Check sheet for the modelled part. Datum: model origin and axes. Units: mm. A direction names the side the tool comes from. Round coordinates to 2 decimals unless told otherwise and drop trailing zeros. Order: outer loops, then holes, each group sorted by start corner. A loop starts at its lowest first (then second) coordinate and runs counter-clockwise, first axis right, second up. Notation, with made-up numbers: (47.25, -38) -> (65.25, -38) arc R31 ccw to (65.25, -9) -> close; hole circle Ø5 at (59.5, 41). An arc over 180 degrees is marked (long way). Answer in a Markdown table with one row per item.
from build123d import *

# Parameters (mm, degrees)
F1_DEPTH = 7
F2_DEPTH = 6
F3_DEPTH = 15


# Not quite as in the source:
# - a feature names something its author has since deleted; it is built from what else it names


with BuildPart() as f1:
    # F0 (on Front) → F1 (new body)
    with BuildSketch(Plane.XZ):
        with BuildLine():
            Line((-4.090710345, -1.9507641112), (-3.3236176952, -1.6008211246))
            Line((-3.3236176952, -1.6008211246), (-3.3236176952, -2.2903047641))
            Line((-3.3236176952, -2.2903047641), (-2.8842022451, -2.2903047641))
            ThreePointArc((-2.8842022451, -2.2903047641), (0.0905031972, 3.0539098469), (3.0652086395, -2.2903047641))
            Line((3.0652086395, -2.2903047641), (3.4491920394, -2.2903047641))
            Line((3.4491920394, -2.2903047641), (3.4491920394, -1.6408955531))
            Line((3.4491920394, -1.6408955531), (4.2162846892, -1.9507641112))
            Line((4.2162846892, -1.9507641112), (4.4794066601, -1.1210844752))
            ThreePointArc((4.4794066601, -1.1210844752), (4.6290079186, 0.2570213688), (4.2328723206, 1.5854162054))
            Line((4.2328723206, 1.5854162054), (5.5865912817, 3.465253188))
            Line((5.5865912817, 3.465253188), (5.5865912817, 5.931237081))
            Line((5.5865912817, 5.931237081), (1.5955031972, 5.931237081))
            Line((1.5955031972, 5.931237081), (4.5903746292, 3.397220974))
            Line((4.5903746292, 3.397220974), (0.0905031972, 3.431237081))
            Line((0.0905031972, 3.431237081), (-4.4093682348, 3.465253188))
            Line((-4.4093682348, 3.465253188), (-1.4144968028, 5.931237081))
            Line((-1.4144968028, 5.931237081), (-5.4144968028, 5.931237081))
            Line((-5.4144968028, 5.931237081), (-5.4144968028, 3.465253188))
            Line((-5.4144968028, 3.465253188), (-4.1709532845, 1.6969049432))
            ThreePointArc((-4.1709532845, 1.6969049432), (-4.6426172218, -0.138188052), (-4.090710345, -1.9507641112))
        make_face()
        Polygon((-3.3236176952, -2.2903047641), (-3.3236176952, -1.6008211246), (-4.090710345, -1.9507641112), (-4.090710345, -2.2903047641), align=None)
        with BuildLine():
            Line((-2.8842022451, -2.2903047641), (-3.3236176952, -2.2903047641))
            Line((-3.3236176952, -2.2903047641), (-4.090710345, -2.2903047641))
            Line((-4.090710345, -2.2903047641), (-4.090710345, -4.9565606735))
            Line((-4.090710345, -4.9565606735), (-3.3236176952, -4.9565606735))
            Line((-3.3236176952, -4.9565606735), (-2.590710345, -4.9565606735))
            Line((-2.590710345, -4.9565606735), (-2.590710345, -3.7436034497))
            Line((-2.590710345, -3.7436034497), (-2.590710345, -2.6957776739))
            ThreePointArc((-2.590710345, -2.6957776739), (-2.7447140714, -2.4982945873), (-2.8842022451, -2.2903047641))
        make_face()
        with BuildLine():
            Line((3.4491920394, -2.2903047641), (3.0652086395, -2.2903047641))
            ThreePointArc((3.0652086395, -2.2903047641), (2.9005872431, -2.5325770701), (2.7162846892, -2.76023612))
            Line((2.7162846892, -2.76023612), (2.7162846892, -3.7879117456))
            Line((2.7162846892, -3.7879117456), (2.7162846892, -4.9565606735))
            Line((2.7162846892, -4.9565606735), (4.2162846892, -4.9497258588))
            Line((4.2162846892, -4.9497258588), (4.2162846892, -2.2903047641))
            Line((4.2162846892, -2.2903047641), (3.4491920394, -2.2903047641))
        make_face()
        with BuildLine():
            ThreePointArc((-2.2823536237, -3.0189388676), (-2.4416925097, -2.8622823851), (-2.590710345, -2.6957776739))
            Line((-2.590710345, -2.6957776739), (-2.590710345, -3.7436034497))
            Line((-2.590710345, -3.7436034497), (-2.2823536237, -3.0189388676))
        make_face()
        Polygon((3.4491920394, -1.6408955531), (3.4491920394, -2.2903047641), (4.2162846892, -2.2903047641), (4.2162846892, -1.9507641112), align=None)
        with BuildLine():
            Line((2.7162846892, -3.7879117456), (2.7162846892, -2.76023612))
            ThreePointArc((2.7162846892, -2.76023612), (2.5594926434, -2.9268342178), (2.39215173, -3.0828332258))
            Line((2.39215173, -3.0828332258), (2.7162846892, -3.7879117456))
        make_face()
        Polygon((1.5955031972, 5.931237081), (-1.4144968028, 5.931237081), (-4.4093682348, 3.465253188), (0.0905031972, 3.431237081), (4.5903746292, 3.397220974), align=None)
    extrude(amount=F1_DEPTH)

    # F0 (on Front) → F2 (cut)
    with BuildSketch(Plane.XZ):
        Polygon((1.5955031972, 5.931237081), (-1.4144968028, 5.931237081), (-4.4093682348, 3.465253188), (0.0905031972, 3.431237081), (4.5903746292, 3.397220974), align=None)
    extrude(amount=F2_DEPTH, mode=Mode.SUBTRACT)

    # F0 (on Front) → F3 (join)
    with BuildSketch(Plane.XZ):
        with BuildLine():
            Line((-2.8842022451, -2.2903047641), (-3.3236176952, -2.2903047641))
            Line((-3.3236176952, -2.2903047641), (-4.090710345, -2.2903047641))
            Line((-4.090710345, -2.2903047641), (-4.090710345, -4.9565606735))
            Line((-4.090710345, -4.9565606735), (-3.3236176952, -4.9565606735))
            Line((-3.3236176952, -4.9565606735), (-2.590710345, -4.9565606735))
            Line((-2.590710345, -4.9565606735), (-2.590710345, -3.7436034497))
            Line((-2.590710345, -3.7436034497), (-2.590710345, -2.6957776739))
            ThreePointArc((-2.590710345, -2.6957776739), (-2.7447140714, -2.4982945873), (-2.8842022451, -2.2903047641))
        make_face()
        with BuildLine():
            Line((3.4491920394, -2.2903047641), (3.0652086395, -2.2903047641))
            ThreePointArc((3.0652086395, -2.2903047641), (2.9005872431, -2.5325770701), (2.7162846892, -2.76023612))
            Line((2.7162846892, -2.76023612), (2.7162846892, -3.7879117456))
            Line((2.7162846892, -3.7879117456), (2.7162846892, -4.9565606735))
            Line((2.7162846892, -4.9565606735), (4.2162846892, -4.9497258588))
            Line((4.2162846892, -4.9497258588), (4.2162846892, -2.2903047641))
            Line((4.2162846892, -2.2903047641), (3.4491920394, -2.2903047641))
        make_face()
    extrude(amount=-F3_DEPTH)


solid = f1.part
Item 1: Cross-section at A-A (y = 0.5). Record the boundary of the cut face in (x, z).
Result sheet:
| item | result |
|---|---|
| outline | (-4.09, -4.96) -> (-2.59, -4.96) -> (-2.59, -2.7) arc R3.5 cw to (-2.88, -2.29) -> (-4.09, -2.29) -> close; (2.72, -4.96) -> (4.22, -4.95) -> (4.22, -2.29) -> (3.07, -2.29) arc R3.5 cw to (2.72, -2.76) -> close |
Item 2: Cross-section at B-B (z = 0.5). Record the boundary of the cut face in (x, y), and give its area (3 significant figures).
Result sheet:
| item | result |
|---|---|
| outline | (-4.6, -7) -> (-3.28, -7) -> (-3.28, 0) -> (-4.6, 0) -> close; (3.46, -7) -> (4.6, -7) -> (4.6, 0) -> (3.46, 0) -> close |
| area | 17.2 mm^2 |
Item 3: Cross-section at C-C (y = -3.25). Record the boundary of the cut face in (x, z), and give its area (3 significant figures).
Result sheet:
| item | result |
|---|---|
| outline | (-5.41, 3.47) -> (-4.17, 1.7) arc R3.51 ccw to (-4.09, -1.95) -> (-4.09, -4.96) -> (-2.59, -4.96) -> (-2.59, -3.74) -> (-2.28, -3.02) arc R3.5 cw (long way) to (2.39, -3.08) -> (2.72, -3.79) -> (2.72, -4.96) -> (4.22, -4.95) -> (4.22, -1.95) -> (4.48, -1.12) arc R3.51 ccw to (4.23, 1.59) -> (5.59, 3.47) -> (5.59, 5.93) -> (1.6, 5.93) -> (4.59, 3.4) -> (-4.41, 3.47) -> (-1.41, 5.93) -> (-5.41, 5.93) -> close |
| area | 41.5 mm^2 |
Item 4: Mould release check, pull along X, two halves, no side actions. Record for faces 6 (the flat face through (-4.8, -3.45, 2.59)), 7 (the flat face through (-3, 4, -4.957)), 8 (the flat face through (0, -6, 4)): pulls with the +X half, pulls with the -X half, needs draft (parallel to the pull), parting line crosses it, or undercut.
Result sheet:
| item | result |
|---|---|
| face 6 | pulls with the -X half |
| face 7 | needs draft |
| face 8 | undercut |
Item 5: Set-up check for faces 1 (the flat face through (2.716, 7, -4)), 2 (the flat face through (4.216, 4, -3)), 3 (the flat face through (3.11, -2.96, 4.65)), 4 (the cylindrical face through (-4.643, -3.451, -0.111)), 5 (the flat face through (-3.5, 7.4, -2.29)): record each of +Z, -Z, +X, -X, +Y, -Y from which the full face is reachable in a straight line by a thin tool's end or side.
Result sheet:
| item | result |
|---|---|
| face 1 | -Z, +Y |
| face 2 | -Z, +X, +Y, -Y |
| face 3 | +Y |
| face 4 | -X, +Y, -Y |
| face 5 | +Z, +X, -X, +Y |
Item 6: Cross-section at D-D (z = 4). Record the boundary of the cut face in (x, y).
Result sheet:
| item | result |
|---|---|
| outline | (-5.41, -7) -> (5.59, -7) -> (5.59, 0) -> (3.88, 0) -> (3.88, -6) -> (-3.76, -6) -> (-3.76, 0) -> (-5.41, 0) -> close |
Item 7: Depth check by flat-ended pin: P1, Ø6.5, axis at x = -1.5, z = 4, coming from the +Y side; P2, Ø6.5, axis at x = 0.09, z = -0.45, coming from the -Y side; P3, Ø0.9, axis at y = 9.5, z = -3, coming from the -X side; P4, Ø1.5, axis at y = 5, z = -2.5, coming from the +X side. Enter the tip coordinate at first touch or a pass-through.
Result sheet:
| item | result |
|---|---|
| P1 | stops at y = 0 |
| P2 | passes through |
| P3 | stops at x = -4.09 |
| P4 | stops at x = 4.22 |
Item 8: Scan lines: line 1 (X direction, y = -3.5, z = -4.5); line 2 (Y direction, x = -2.75, z = 5); line 3 (Z direction, x = -3.25, y = 6.25). Record each from-to range of solid material in increasing order. Write a range as [from, to].
Result sheet:
| item | result |
|---|---|
| line 1 | x = [-4.09, -2.59], [2.72, 4.22] |
| line 2 | y = [-7, 0] |
| line 3 | z = [-4.96, -2.29] |
